Source: CAD feature listing. Evaluate the final solid. Frame: model axes, mm. A direction names the side the tool comes from. Round coordinates to 2 decimals unless told otherwise and drop trailing zeros. Order: outer loops, then holes, each group sorted by start corner. A loop starts at its lowest first (then second) coordinate and runs counter-clockwise, first axis right, second up. Notation, with made-up numbers: (-14, -23.5) -> (0, -23.5) arc R28 ccw to (0, 2.5) -> close; hole circle Ø3 at (9.25, -17.75). An arc over 180 degrees is marked (long way). One line per item, written item: value. Start each with the question number.
1) Section A-A (y = 0). Return the cut outline in (x, z), and give its area (3 significant figures).
2) Pin query (flat end, axial travel): P1, Ø2.5, axis at x = 0, z = 8, coming from the +Y side; P2, Ø4, axis at y = 5, z = -2.5, coming from the +X side; P3, Ø1.5, axis at x = 11.5, z = 2, coming from the +Y side. Return the tip coordinate at first contact, or that it passes through.
3) Section D-D (y = -15.5). Return the cut outline in (x, z), and give its area (3 significant figures).
4) Mould query, pull axis Y, two halves, no side actions, for faces 6 (the face through (-7, 18, 3.5)), 7 (the face through (-4.769, -21.477, 3.993)), 8 (the face through (-1.08, -4.88, 3.4)). Classes: pulls with the +Y half, pulls with the -Y half, needs draft (parallel to the pull), parting line crosses it, or undercut.
5) Ray query, L1, parallel to Z at x = 0, y = 10; L2, parallel to Z at x = -14, y = -2; L3, parallel to Y at x = -3, z = 10.5. Return the intervals inside material, ascending.
6) Section B-B (x = 0). State how many separate pieces and enclosed holes the cut face has, and give its area (4 significant figures).
7) Section C-C (z = 5.25). Return the cut outline in (x, y), and give its area (3 significant figures).
8) Reachability of faces 1 (the face through (-0.325, 8.579, 6.536)), 2 (the face through (-4.769, -21.477, -3.993)), 3 (the face through (5, -5, -4.5)), 4 (the face through (9, -9, 4.5)), 5 (the face through (8.767, -16.856, 0.049)) from +Z, -Z, +X, -X, +Y, -Y: full face, straight path, thin tool, end or side. Return the list, or none.
```python
from build123d import *

# Parameters (mm, degrees)
F0_R     = 19
F0_R_2   = 5
F1_DEPTH = 3.5
F2_R     = 22
F2_R_2   = 5
F3_DEPTH = 1
F5_R     = 12.5
F5_R_2   = 5
F6_DEPTH = 7
F7_SIZE  = 1
F8_R     = 1.5
F9_DEPTH = 22.001


with BuildPart() as f1:
    # F0 (on Top) → F1 (new body, symmetric)
    with BuildSketch(Plane.XY):
        Circle(F0_R)
        Circle(F0_R_2, mode=Mode.SUBTRACT)
    extrude(amount=F1_DEPTH, both=True)

    # F2 (on face) → F3 (join)
    with BuildSketch(Plane.XY.offset(3.5)):
        Circle(F2_R)
        Circle(F2_R_2, mode=Mode.SUBTRACT)
    extrude(amount=F3_DEPTH)

    # F4: F1 across plane


with BuildPart() as f1_1:
    add(f1.part)
    add(f1.part.mirror(Plane.XY))

    # F5 (on face) → F6 (join)
    with BuildSketch(Plane.XY.offset(4.5)):
        Circle(F5_R)
        Circle(F5_R_2, mode=Mode.SUBTRACT)
    extrude(amount=F6_DEPTH)

    # F7
    f7_edges = [f1_1.edges().sort_by_distance(p)[0] for p in [
        (-12.5, 0, 11.5),
        (-5, 0, 11.5),
        (-5, 0, -4.5),
    ]]
    chamfer(f7_edges, length=F7_SIZE)

    # F8 (on Front) → F9 (cut, through all)
    with BuildSketch(Plane.XZ):
        with Locations((0, 8)):
            Circle(F8_R)
    extrude(amount=-F9_DEPTH, mode=Mode.SUBTRACT)


solid = f1_1.part
```
Findings:
1. outline: (-22, -4.5) -> (-6, -4.5) -> (-5, -3.5) -> (-5, 10.5) -> (-6, 11.5) -> (-11.5, 11.5) -> (-12.5, 10.5) -> (-12.5, 4.5) -> (-22, 4.5) -> (-22, 3.5) -> (-19, 3.5) -> (-19, -3.5) -> (-22, -3.5) -> close; (5, -3.5) -> (6, -4.5) -> (22, -4.5) -> (22, -3.5) -> (19, -3.5) -> (19, 3.5) -> (22, 3.5) -> (22, 4.5) -> (12.5, 4.5) -> (12.5, 10.5) -> (11.5, 11.5) -> (6, 11.5) -> (5, 10.5) -> close
1. area: 366 mm2
2. P1: y = -4.84
2. P2: x = 21.76
2. P3: y = 15.67
3. outline: (-15.61, -4.5) -> (15.61, -4.5) -> (15.61, -3.5) -> (10.99, -3.5) -> (10.99, 3.5) -> (15.61, 3.5) -> (15.61, 4.5) -> (-15.61, 4.5) -> (-15.61, 3.5) -> (-10.99, 3.5) -> (-10.99, -3.5) -> (-15.61, -3.5) -> close
3. area: 216 mm2
4. face 6: needs draft
4. face 7: parting line crosses it
4. face 8: undercut
5. L1: -4.5 to 6.5, 9.5 to 11.5
5. L2: -4.5 to 4.5
5. L3: -12.13 to -4, 4 to 12.13
6. separate pieces: 3
6. enclosed holes: 0
6. area: 343.5 mm2
7. outline: circle Ø25 at (0, 0); hole circle Ø10 at (0, 0)
7. area: 412 mm2
8. face 1: +Y
8. face 2: +Z, -Z
8. face 3: -Z, +X, -X, +Y, -Y
8. face 4: +Z
8. face 5: none
